Work out the finished part from the listing and answer in its coordinate system (mm). Face numbers are marked on the shaded views. A direction names the side the tool comes from. Give positions to 0.01 mm unless a question says otherwise; leave off trailing zeros. Loops run counter-clockwise (first coordinate to the right, second up) from the corner with the lowest first, then second, coordinate; pieces in that order, holes last. Notation, with made-up numbers: (68, 43.5) -> (94, 43.5) arc R21 cw to (94, 60.5) -> close; hole circle Ø10 at (-37.75, 30.5). An arc over 180 degrees is marked (long way). Answer as CSV lines item,"result". Start each with the question number.
1. Find the intervals of material crossed by line 1 along X through (y, z) = (1.5, 15.5); line 2 along Z through (x, y) = (21, 0.6); line 3 along X through (y, z) = (17.25, 19), in increasing order.
2. Find section C-C, the plane x = 14. Give the vertices of the cut face in (y, z), and give its area (3 significant figures).
3. A tool of negligible diameter and unlimited length cuts with its end or side. For the marked faces 1, 2, 3 and 4, from which of +Z, -Z, +X, -X, +Y, -Y can it reach the whole face along a straight path? Write none if from no direction.
4. Determine the mould class of the marked faces 5, 6 and 7 for opening direction X: +X half, -X half, draft (parallel to the pull), parting line (faces both ways), or undercut.
5. Flat-ended cylindrical pins translate along their axes: pin 1 Ø2.5 at (x, z) = (-22, -2) entering from +Y; pin 2 Ø5 at (y, z) = (14.5, 13.5) entering from +X; pin 3 Ø2 at (y, z) = (17.5, 14) entering from -X. Find the tip coordinate at first contact, or state that the pin passes through.
6. Find section B-B, the plane x = 21. Give the vertices of the cut face in (y, z).
7. Find section A-A, the plane y = 12. Give the vertices of the cut face in (x, z).
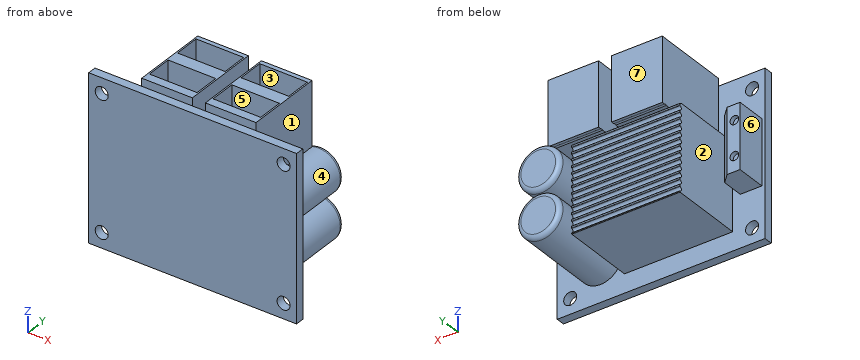
from build123d import *

# Parameters (mm, degrees)
SKETCH1_W           = 48
SKETCH1_H           = 38
SKETCH1_R           = 1.5
BOSS_EXTRUDE1_DEPTH = 2
SKETCH2_W           = 11.7
SKETCH2_H           = 14.8
BOSS_EXTRUDE2_DEPTH = 18
SKETCH3_W           = 11
SKETCH3_H           = 6
CUT_EXTRUDE1_DEPTH  = 13
SKETCH4_W           = 11
SKETCH4_H           = 11
BOSS_EXTRUDE3_DEPTH = 2
SKETCH5_W           = 11
SKETCH5_H           = 11
BOSS_EXTRUDE4_DEPTH = 2
SKETCH6_W           = 25
SKETCH6_H           = 20
BOSS_EXTRUDE5_DEPTH = 17
SKETCH7_R           = 0.5
CUT_EXTRUDE2_DEPTH  = 41.536312966
FILLET1_R           = 0.1
SKETCH8_R           = 5
BOSS_EXTRUDE6_DEPTH = 20
FILLET2_R           = 1
SKETCH9_W           = 5
SKETCH9_H           = 15
BOSS_EXTRUDE7_DEPTH = 7
CHAMFER1_SIZE       = 2
SKETCH10_R          = 1
CUT_EXTRUDE3_DEPTH  = 1


with BuildPart() as part:
    # Sketch1 → Boss-Extrude1 (new body)
    with BuildSketch(Plane(origin=(0, 0, 0), x_dir=(1, 0, 0), z_dir=(0, 1, 0))):
        Rectangle(SKETCH1_W, SKETCH1_H)
        with Locations((-21, 15.5)):
            Circle(SKETCH1_R, mode=Mode.SUBTRACT)
        with Locations((-21, -15.5)):
            Circle(SKETCH1_R, mode=Mode.SUBTRACT)
        with Locations((21, -15.5)):
            Circle(SKETCH1_R, mode=Mode.SUBTRACT)
        with Locations((21, 15.5)):
            Circle(SKETCH1_R, mode=Mode.SUBTRACT)
    extrude(amount=BOSS_EXTRUDE1_DEPTH)

    # Sketch2 → Boss-Extrude2 (add)
    with BuildSketch(Plane(origin=(0, 2, 0), x_dir=(1, 0, 0), z_dir=(0, 1, 0))):
        with Locations((-7.35, -13.4)):
            Rectangle(SKETCH2_W, SKETCH2_H)
    boss_extrude2 = extrude(amount=BOSS_EXTRUDE2_DEPTH)

    # Sketch3 → Cut-Extrude1 (cut)
    with BuildSketch(Plane.XY.offset(20.8)):
        with Locations((-7.35, 16)):
            Rectangle(SKETCH3_W, SKETCH3_H)
        with Locations((-7.35, 7)):
            Rectangle(SKETCH3_W, SKETCH3_H)
    cut_extrude1 = extrude(amount=-CUT_EXTRUDE1_DEPTH, mode=Mode.SUBTRACT)

    # Sketch4 → Boss-Extrude3 (add)
    with BuildSketch(Plane(origin=(0, 13, 0), x_dir=(1, 0, 0), z_dir=(0, 1, 0))):
        with Locations((-7.35, -13.3)):
            Rectangle(SKETCH4_W, SKETCH4_H)
    boss_extrude3 = extrude(amount=BOSS_EXTRUDE3_DEPTH)

    # Sketch5 → Boss-Extrude4 (add)
    with BuildSketch(Plane(origin=(0, 4, 0), x_dir=(1, 0, 0), z_dir=(0, 1, 0))):
        with Locations((-7.35, -13.3)):
            Rectangle(SKETCH5_W, SKETCH5_H)
    boss_extrude4 = extrude(amount=BOSS_EXTRUDE4_DEPTH)

    # Mirror1: Boss-Extrude2, Cut-Extrude1, Boss-Extrude3, Boss-Extrude4 across plane
    add(boss_extrude2.mirror(Plane(origin=(0, 0, 0), x_dir=(0, 0, 1), z_dir=(1, 0, 0))))
    add(cut_extrude1.mirror(Plane(origin=(0, 0, 0), x_dir=(0, 0, 1), z_dir=(1, 0, 0))), mode=Mode.SUBTRACT)
    add(boss_extrude3.mirror(Plane(origin=(0, 0, 0), x_dir=(0, 0, 1), z_dir=(1, 0, 0))))
    add(boss_extrude4.mirror(Plane(origin=(0, 0, 0), x_dir=(0, 0, 1), z_dir=(1, 0, 0))))

    # Sketch6 → Boss-Extrude5 (add)
    with BuildSketch(Plane(origin=(0, 2, 0), x_dir=(1, 0, 0), z_dir=(0, 1, 0))):
        with Locations((-4.036312966, 4.7)):
            Rectangle(SKETCH6_W, SKETCH6_H)
    extrude(amount=BOSS_EXTRUDE5_DEPTH)

    # Sketch7 → Cut-Extrude2 (cut, through all)
    with BuildSketch(Plane.ZY.offset(16.536312966)):
        with Locations((-13.901253827, 19)):
            Circle(SKETCH7_R)
        with Locations((-12.401253827, 19)):
            Circle(SKETCH7_R)
        with Locations((-10.901253827, 19)):
            Circle(SKETCH7_R)
        with Locations((-9.401253827, 19)):
            Circle(SKETCH7_R)
        with Locations((-7.901253827, 19)):
            Circle(SKETCH7_R)
        with Locations((-6.401253827, 19)):
            Circle(SKETCH7_R)
        with Locations((-4.901253827, 19)):
            Circle(SKETCH7_R)
        with Locations((-3.401253827, 19)):
            Circle(SKETCH7_R)
        with Locations((-1.901253827, 19)):
            Circle(SKETCH7_R)
        with Locations((-0.401253827, 19)):
            Circle(SKETCH7_R)
        with Locations((1.098746173, 19)):
            Circle(SKETCH7_R)
        with Locations((2.598746173, 19)):
            Circle(SKETCH7_R)
        with Locations((4.098746173, 19)):
            Circle(SKETCH7_R)
        with Locations((5.598746173, 19)):
            Circle(SKETCH7_R)
    extrude(amount=-CUT_EXTRUDE2_DEPTH, mode=Mode.SUBTRACT)

    # Fillet1
    fillet1_edges = [part.edges().sort_by_distance(p)[0] for p in [
        (-4.036312966, 19, -14.7),
        (-4.036312966, 19, -13.401253827),
        (-4.036312966, 19, -14.401253827),
        (-4.036312966, 19, -11.901253827),
        (-4.036312966, 19, -12.901253827),
        (-4.036312966, 19, -10.401253827),
        (-4.036312966, 19, -11.401253827),
        (-4.036312966, 19, -8.901253827),
        (-4.036312966, 19, -9.901253827),
        (-4.036312966, 19, -7.401253827),
        (-4.036312966, 19, -8.401253827),
        (-4.036312966, 19, -5.901253827),
        (-4.036312966, 19, -6.901253827),
        (-4.036312966, 19, -4.401253827),
        (-4.036312966, 19, -5.401253827),
        (-4.036312966, 19, -2.901253827),
        (-4.036312966, 19, -3.901253827),
        (-4.036312966, 19, -1.401253827),
        (-4.036312966, 19, -2.401253827),
        (-4.036312966, 19, 0.098746173),
        (-4.036312966, 19, -0.901253827),
        (-4.036312966, 19, 1.598746173),
        (-4.036312966, 19, 0.598746173),
        (-4.036312966, 19, 3.098746173),
        (-4.036312966, 19, 2.098746173),
        (-4.036312966, 19, 4.598746173),
        (-4.036312966, 19, 3.598746173),
        (-4.036312966, 19, 5.098746173),
    ]]
    fillet(fillet1_edges, radius=FILLET1_R)

    # Sketch8 → Boss-Extrude6 (add)
    with BuildSketch(Plane(origin=(0, 2, 0), x_dir=(1, 0, 0), z_dir=(0, 1, 0))):
        with Locations((14, 10)):
            Circle(SKETCH8_R)
        with Locations((14, -0.5)):
            Circle(SKETCH8_R)
    extrude(amount=BOSS_EXTRUDE6_DEPTH)

    # Fillet2
    fillet2_edges = [part.edges().sort_by_distance(p)[0] for p in [
        (9, 22, -10),
        (9, 22, 0.5),
    ]]
    fillet(fillet2_edges, radius=FILLET2_R)

    # Sketch9 → Boss-Extrude7 (add)
    with BuildSketch(Plane(origin=(0, 2, 0), x_dir=(1, 0, 0), z_dir=(0, 1, 0))):
        with Locations((-20.760712337, -0.5)):
            Rectangle(SKETCH9_W, SKETCH9_H)
    extrude(amount=BOSS_EXTRUDE7_DEPTH)

    # Chamfer1
    chamfer1_edges = [part.edges().sort_by_distance(p)[0] for p in [
        (-18.260712337, 9, 0.5),
    ]]
    chamfer(chamfer1_edges, length=CHAMFER1_SIZE)

    # Sketch10 → Cut-Extrude3 (cut)
    with BuildSketch(Plane(origin=(0, 9, 0), x_dir=(1, 0, 0), z_dir=(0, 1, 0))):
        with Locations((-21.952606412, 3.5)):
            Circle(SKETCH10_R)
        with Locations((-21.952606412, -4.5)):
            Circle(SKETCH10_R)
    extrude(amount=-CUT_EXTRUDE3_DEPTH, mode=Mode.SUBTRACT)


solid = part.part
Resolved:
1,line 1,"x = -24 to -22.5, -19.5 to 19.5, 22.5 to 24"
1,line 2,"z = -19 to -17, -14 to 14, 17 to 19"
1,line 3,"x = -13.2 to -12.85, -1.85 to -1.5, 1.5 to 1.85, 12.85 to 13.2"
2,outline,"(0, -19) -> (2, -19) -> (2, -15) -> (21, -15) arc R1 ccw to (22, -14) -> (22, -6) arc R1 ccw to (21, -5) -> (2, -5) -> (2, -4.5) -> (21, -4.5) arc R1 ccw to (22, -3.5) -> (22, 4.5) arc R1 ccw to (21, 5.5) -> (2, 5.5) -> (2, 19) -> (0, 19) -> close"
2,area,"475 mm^2"
3,face 1,"+Z, +X, +Y"
3,face 2,"+Z, -Z, +Y"
3,face 3,"+Z"
3,face 4,"+Y"
4,face 5,"undercut"
4,face 6,"-X half"
4,face 7,"draft"
5,pin 1,"stops at y = 9"
5,pin 2,"stops at x = 13.2"
5,pin 3,"stops at x = -13.2"
6,outline,"(0, -19) -> (2, -19) -> (2, -17) -> (0, -17) -> close; (0, -14) -> (2, -14) -> (2, 14) -> (0, 14) -> close; (0, 17) -> (2, 17) -> (2, 19) -> (0, 19) -> close"
7,outline,"(-16.54, -14.7) -> (8.46, -14.7) -> (8.46, 5.3) -> (-16.54, 5.3) -> close; (-13.2, 6) -> (-1.5, 6) -> (-1.5, 20.8) -> (-13.2, 20.8) -> close; (1.5, 6) -> (13.2, 6) -> (13.2, 20.8) -> (1.5, 20.8) -> close; circle Ø10 at (14, -10); circle Ø10 at (14, 0.5)"
